The listing builds one solid part. Answer for the finished solid, in the listing's coordinates (mm). Coordinates: 2 decimals unless noted, no trailing zeros. Order: outer loops, then holes, each group sorted by start corner. A loop starts at its lowest first (then second) coordinate and runs counter-clockwise, first axis right, second up. Notation, with made-up numbers: M 52.25,81.5 L 97.25,81.5 A15 ccw 97.25,92.5 Z; hole C 45,75.5 d4. An arc over 180 degrees is marked long. One line per item, written item: value. Start each with the question number.
Q1. The part is cut by section A-A on z = -9.5. Give the vertices of the cut face in (x, y), then the cut area to 3 significant figures.
Q2. Each of these flat-tipped pins is pushed along its axis until it touches: pin 1 Ø13 at (x, y) = (-6, -2.5) entering from -Z; pin 2 Ø2 at (x, y) = (8, 2) entering from -Z. Where does it stop, or does it pass through?
Q3. The part is cut by section B-B on x = -8. Give the vertices of the cut face in (y, z).
Q4. Straight lines are drawn through the part: line 1 along Z through (x, y) = (4, 10.25); line 2 along Z through (x, y) = (-11.5, -5.25); line 3 along X through (y, z) = (-10, 19.5). For each, find the intervals that lie inside material, in ascending order. Write a range as [from, to].
Q5. The part is cut by section D-D on y = -10.5. Give the vertices of the cut face in (x, z), then the cut area to 3 significant figures.
```python
from build123d import *

# Parameters (mm, degrees)
SKETCH_1_W      = 26
SKETCH_1_H      = 26
EXTRUDE_1_DEPTH = 21
FILLET_1_R      = 2
SKETCH_2_R      = 0.5
EXTRUDE_2_DEPTH = 12


with BuildPart() as part:
    # 草图1 → 凸台-拉伸1 (new body)
    with BuildSketch(Plane.XY):
        Rectangle(SKETCH_1_W, SKETCH_1_H)
    extrude(amount=EXTRUDE_1_DEPTH)

    # 圆角1
    fillet_1_edges = [part.edges().sort_by_distance(p)[0] for p in [
        (13, 0, 21),
        (0, 13, 21),
        (-13, 0, 21),
        (0, -13, 21),
    ]]
    fillet(fillet_1_edges, radius=FILLET_1_R)

    # 草图2 → 凸台-拉伸2 (add)
    with BuildSketch(Plane(origin=(0, 0, 0), x_dir=(-1, 0, 0), z_dir=(0, 0, -1))):
        with Locations(Location((-8, 8, 0), (0, 0, 180))):
            Circle(SKETCH_2_R)
        with Locations(Location((-8, 0, 0), (0, 0, 180))):
            Circle(SKETCH_2_R)
        with Locations(Location((-8, -8, 0), (0, 0, 180))):
            Circle(SKETCH_2_R)
        with Locations(Location((8, -8, 0), (0, 0, 180))):
            Circle(SKETCH_2_R)
        with Locations(Location((8, 8, 0), (0, 0, 180))):
            Circle(SKETCH_2_R)
    extrude(amount=EXTRUDE_2_DEPTH)


solid = part.part
```
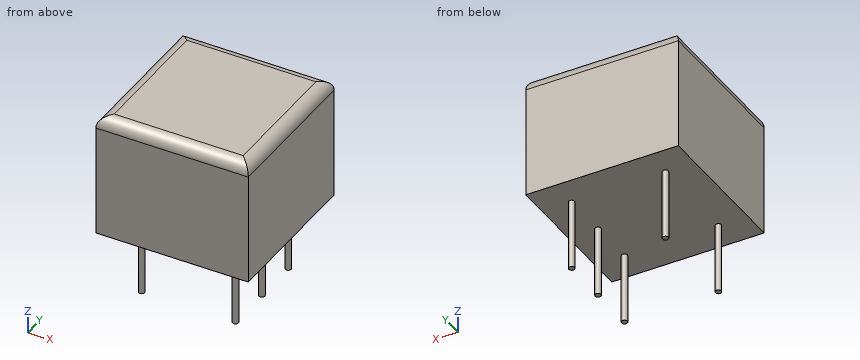
Output:
1. outline: C -8,-8 d1; C -8,8 d1; C 8,-8 d1; C 8,0 d1; C 8,8 d1
1. area: 3.93 mm^2
2. pin 1: stops at z = -12
2. pin 2: stops at z = 0
3. outline: M -13,0 L -8.5,0 L -8.5,-12 L -7.5,-12 L -7.5,0 L 7.5,0 L 7.5,-12 L 8.5,-12 L 8.5,0 L 13,0 L 13,19 A2 ccw 11,21 L -11,21 A2 ccw -13,19 Z
4. line 1: z = [0, 21]
4. line 2: z = [0, 20.94]
4. line 3: x = [-12.94, 12.94]
5. outline: M -13,0 L 13,0 L 13,19 A2 ccw 11,21 L -11,21 A2 ccw -13,19 Z
5. area: 544 mm^2
